Build history of the part. All positions in model axes, mm. Face numbers are marked on the shaded views. A direction names the side the tool comes from. Round coordinates to 2 decimals unless told otherwise and drop trailing zeros. Loops run counter-clockwise (first coordinate to the right, second up) from the corner with the lowest first, then second, coordinate; pieces in that order, holes last. Notation, with made-up numbers: (35.5, 22.25) - (86.5, 22.25) arc R23 cw to (86.5, 49.25) - close; hole circle Ø11 at (-14, -18.5). An arc over 180 degrees is marked (long way). Use a Markdown table: item, result.
from build123d import *

# Parameters (mm, degrees)
SKETCH1_W                = 12
SKETCH1_H                = 22
BOSS_EXTRUDE1_DEPTH      = 5
BOSS_EXTRUDE2_DEPTH      = 3
BOSS_EXTRUDE2_DEPTH_BACK = 25
SKETCH2_R                = 4.877853957
CUT_EXTRUDE1_DEPTH       = 16
CUT_EXTRUDE1_DEPTH_BACK  = 16
SKETCH4_R                = 0.5


with BuildPart() as part:
    # Sketch1 → Boss-Extrude1 (new body)
    with BuildSketch(Plane(origin=(0, 0, 0), x_dir=(1, 0, 0), z_dir=(0, 1, 0))):
        with Locations((6.730337079, 0)):
            Rectangle(SKETCH1_W, SKETCH1_H)
    extrude(amount=BOSS_EXTRUDE1_DEPTH)

    # Sketch2 → Boss-Extrude2 (add, two sides: drawn at the far end of the back side and taken through both)
    with BuildSketch(Plane.XY.offset(11).offset(-BOSS_EXTRUDE2_DEPTH_BACK)):
        with BuildLine():
            Line((-3.78803397, 16.755707913), (17.248708128, 16.755707913))
            ThreePointArc((17.248708128, 16.755707913), (23.126562084, 10.877853957), (17.248708128, 5))
            Line((17.248708128, 5), (-3.78803397, 5))
            ThreePointArc((-3.78803397, 5), (-9.665887927, 10.877853957), (-3.78803397, 16.755707913))
        make_face()
        with Locations((17.248708128, 10.877853957)):
            Circle(SKETCH2_R, mode=Mode.SUBTRACT)
        with Locations((6.730337079, 10.877853957)):
            Circle(SKETCH2_R, mode=Mode.SUBTRACT)
        with Locations((-3.78803397, 10.877853957)):
            Circle(SKETCH2_R, mode=Mode.SUBTRACT)
    extrude(amount=BOSS_EXTRUDE2_DEPTH + BOSS_EXTRUDE2_DEPTH_BACK)

    # Sketch4 → Cut-Extrude1 (cut, two sides: drawn at the far end of the back side and taken through both)
    with BuildSketch(Plane(origin=(6.730337079, 0, 0), x_dir=(0, 0, -1), z_dir=(1, 0, 0)).offset(-CUT_EXTRUDE1_DEPTH_BACK)):
        with Locations((-9.12, 10.877853957)):
            Circle(SKETCH4_R)
    extrude(amount=CUT_EXTRUDE1_DEPTH + CUT_EXTRUDE1_DEPTH_BACK, mode=Mode.SUBTRACT)


solid = part.part
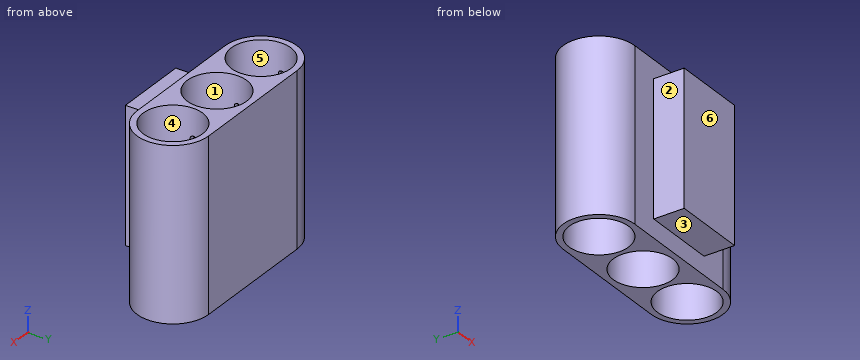
Q1. Which spindle directions (+Z, -Z, +X, -X, +Y, -Y) get a long thin tool onto all of the face, cutting with end or side? Do the marked faces 1 and 2. Say none if no direction does.
Results found:
| item | result |
|---|---|
| face 1 | +Z, -Z |
| face 2 | +Z, -Z, -X, -Y |
Q2. Cut at D-D, the plane z = 0.5. List the corners of the cut face in (x, y), plus the area to 3 significant figures.
Results found:
| item | result |
|---|---|
| outline | (-3.79, 5) - (0.73, 5) - (0.73, 0) - (12.73, 0) - (12.73, 5) - (17.25, 5) arc R5.88 ccw to (17.25, 16.76) - (-3.79, 16.76) arc R5.88 ccw to start; hole circle Ø9.76 at (-3.79, 10.88); hole circle Ø9.76 at (6.73, 10.88); hole circle Ø9.76 at (17.25, 10.88) |
| area | 192 mm2 |
Q3. Cut at B-B, the plane x = 4.5. List the corners of the cut face in (y, z), plus the area to 3 significant figures.
Results found:
| item | result |
|---|---|
| outline | (0, -11) - (5, -11) - (5, -14) - (6.54, -14) - (6.54, 14) - (5, 14) - (5, 11) - (0, 11) - close; (15.22, -14) - (16.76, -14) - (16.76, 14) - (15.22, 14) - close |
| area | 196 mm2 |
Q4. Pull direction Y, two halves, no side cores. Call the marked faces 3, 4, 5 and 6: pulls with the +Y half, pulls with the -Y half, needs draft (parallel to the pull), parting line crosses it, or undercut.
Results found:
| item | result |
|---|---|
| face 3 | needs draft |
| face 4 | undercut |
| face 5 | undercut |
| face 6 | pulls with the -Y half |
Q5. Drop flat-ended pins along their axis: pin 1 (5.5 mm diameter, centred on x = 8.5, y = 1.5, fed in from +Z); pin 2 (4 mm diameter, centred on y = 3.5, z = -5, fed in from -X); pin 3 (8 mm diameter, centred on y = 4.5, z = -10, fed in from -X). Give the stop position or say it passes through.
Results found:
| item | result |
|---|---|
| pin 1 | stops at z = 11 |
| pin 2 | stops at x = -6.16 |
| pin 3 | stops at x = -9.16 |
Q6. Probe line 1 (Y direction, x = 12.25, z = 9.12); line 2 (X direction, y = 11.25, z = -8); line 3 (X direction, y = 15, z = -3). List the from-to ranges inside material, lowest first.
Results found:
| item | result |
|---|---|
| line 1 | y = 0 to 10.38, 11.38 to 16.76 |
| line 2 | x = -9.65 to -8.65, 1.08 to 1.87, 11.59 to 12.39, 22.11 to 23.11 |
| line 3 | x = -7.98 to -6.4, -1.18 to 4.12, 9.34 to 14.64, 19.86 to 21.44 |
Q7. Cut at C-C, the plane y = 12.5. List the corners of the cut face in (x, z), plus the area to 3 significant figures.
Results found:
| item | result |
|---|---|
| outline | (-9.44, -14) - (-8.39, -14) - (-8.39, 14) - (-9.44, 14) - close; (0.81, -14) - (2.13, -14) - (2.13, 14) - (0.81, 14) - close; (11.33, -14) - (12.65, -14) - (12.65, 14) - (11.33, 14) - close; (21.85, -14) - (22.9, -14) - (22.9, 14) - (21.85, 14) - close |
| area | 133 mm2 |
Q8. Cut at A-A, the plane z = 9.12. List the corners of the cut face in (x, y).
Results found:
| item | result |
|---|---|
| outline | (-3.79, 5) - (0.73, 5) - (0.73, 0) - (12.73, 0) - (12.73, 5) - (17.25, 5) arc R5.88 ccw to (17.25, 16.76) - (-3.79, 16.76) arc R5.88 ccw to start; hole (-9.27, 10.38) - (-8.64, 10.38) arc R4.88 ccw to (1.06, 10.38) - (1.88, 10.38) arc R4.88 ccw to (11.58, 10.38) - (12.4, 10.38) arc R4.88 ccw to (22.1, 10.38) - (22.73, 10.38) - (22.73, 11.38) - (22.1, 11.38) arc R4.88 ccw to (12.4, 11.38) - (11.58, 11.38) arc R4.88 ccw to (1.88, 11.38) - (1.06, 11.38) arc R4.88 ccw to (-8.64, 11.38) - (-9.27, 11.38) - close |
